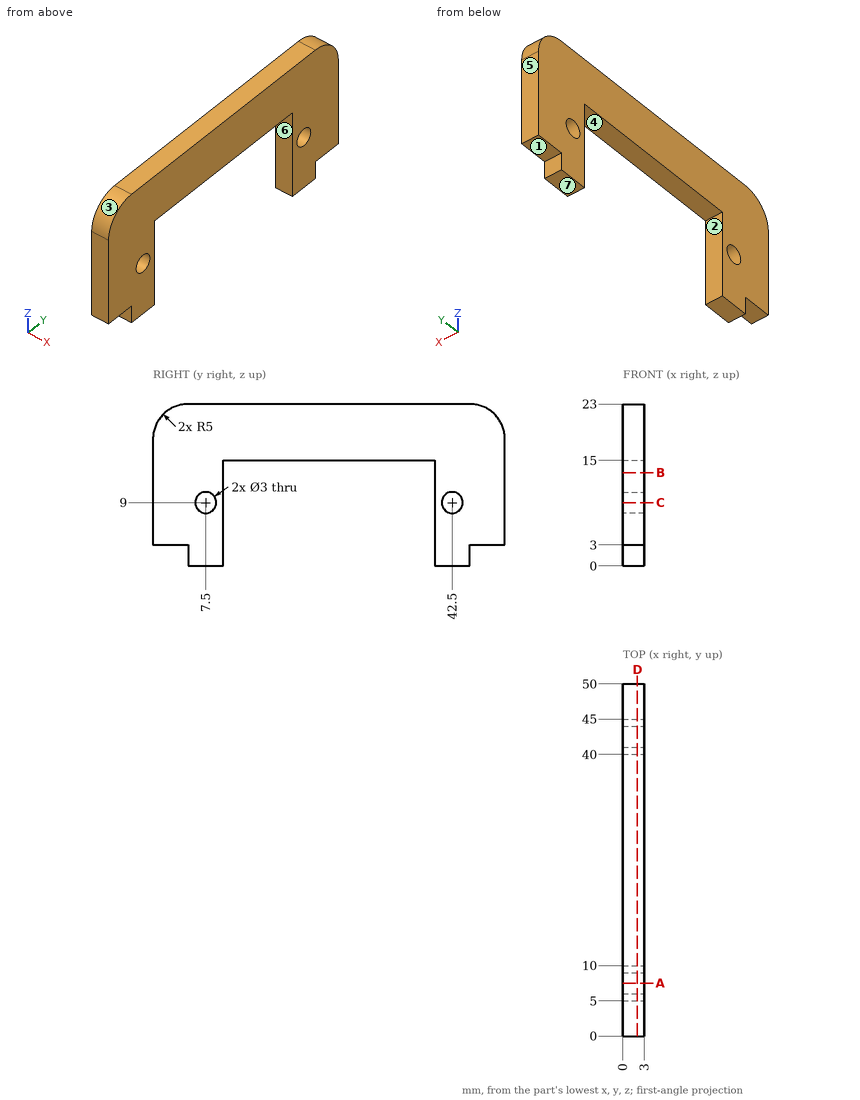
Answer from the drawing. Dimensions are ordinates in mm from the lowest x, y and z of the part. A direction names the side the tool comes from. Round coordinates to 2 decimals unless told otherwise and drop trailing zeros. Write each loop counter-clockwise with the first axis right and the second up, starting at its lowest first coordinate (ties: lowest second). Pieces come first, ordered by that corner, then holes. Notation, with made-up numbers: M 49.5,82 L 63.5,82 A19 cw 63.5,113 Z; hole C 57.5,47.25 d7. An arc over 180 degrees is marked long. Write each question's results on one line, items separated by ' | '. Start each with the question number.
Item 1: Find section A-A on y = 7.5. Write down the section's boundary in (x, z), and give its area (3 significant figures).
Item 2: Find section D-D on x = 2.05. Write down the section's boundary in (y, z).
Item 3: Given pin 1 Ø1.5 at (x, z) = (1.5, 1) entering from +Y; pin 2 Ø1.5 at (x, y) = (2, 1.5) entering from -Z; pin 3 Ø1.5 at (x, z) = (1.5, 1.5) entering from -Y, each flat-ended and moving along its own axis, determine where each tip first touches the part or whether it passes through.
Item 4: Find section B-B on z = 13.25. Write down the section's boundary in (x, y), and give its area (3 significant figures).
Item 5: Find section C-C on z = 9. Write down the section's boundary in (x, y).
Item 6: Which of the six approach directions +Z, -Z, +X, -X, +Y, -Y give full straight-line access (tool end or side, diameter ignored) to the marked faces 1, 2 and 3?
Item 7: Straight lines are drawn through the part: probe 1 along Y at (x, z) = (1.8, 9); probe 2 along Y at (x, z) = (1.8, 13); probe 3 along Y at (x, z) = (2, 7.75). For each, find the intervals that lie inside material, in ascending order.
Item 8: The mould has two halves that part along Y. Classify the marked faces 4, 5, 6 and 7: +Y half, -Y half, draft (parallel to the pull), parting line (faces both ways), or undercut.
Answer block:
1) outline: M 0,0 L 3,0 L 3,7.5 L 0,7.5 Z; M 0,10.5 L 3,10.5 L 3,23 L 0,23 Z | area: 60.0 mm²
2) outline: M 0,3 L 5,3 L 5,0 L 10,0 L 10,15 L 40,15 L 40,0 L 45,0 L 45,3 L 50,3 L 50,18 A5 ccw 45,23 L 5,23 A5 ccw 0,18 Z; hole C 7.5,9 d3; hole C 42.5,9 d3
3) pin 1: stops at y = 45 | pin 2: stops at z = 3 | pin 3: stops at y = 5
4) outline: M 0,0 L 3,0 L 3,10 L 0,10 Z; M 0,40 L 3,40 L 3,50 L 0,50 Z | area: 60.0 mm²
5) outline: M 0,0 L 3,0 L 3,6 L 0,6 Z; M 0,9 L 3,9 L 3,10 L 0,10 Z; M 0,40 L 3,40 L 3,41 L 0,41 Z; M 0,44 L 3,44 L 3,50 L 0,50 Z
6) face 1: -Z, +X, -X, +Y | face 2: -Z, +X, -X | face 3: +Z, +X, -X, -Y
7) probe 1: y = 0 to 6, 9 to 10, 40 to 41, 44 to 50 | probe 2: y = 0 to 10, 40 to 50 | probe 3: y = 0 to 6.67, 8.33 to 10, 40 to 41.67, 43.33 to 50
8) face 4: undercut | face 5: +Y half | face 6: undercut | face 7: draft
